from build123d import *

# Parameters (mm, degrees)
F0_W     = 14
F0_H     = 10
F0_W_2   = 6
F0_H_2   = 6
F1_DEPTH = 3
F2_DEPTH = 9


with BuildPart() as f1:
    # F0 (on Front) → F1 (new body)
    with BuildSketch(Plane.XZ):
        with Locations((-3, 0)):
            Rectangle(F0_W, F0_H)
        with Locations((-3.5, 0)):
            Rectangle(F0_W_2, F0_H_2, mode=Mode.SUBTRACT)
    extrude(amount=F1_DEPTH)

    # F0 (on Front) → F2 (join)
    with BuildSketch(Plane.XZ):
        with Locations((7, 0)):
            Rectangle(F0_W_2, F0_H)
    extrude(amount=F2_DEPTH)


solid = f1.part
Could you check a few things on this model? Use its own coordinates, in mm. A direction names the side the tool comes from. Give positions to 0.01 mm unless a question says otherwise; leave off trailing zeros. Write each loop counter-clockwise with the first axis right and the second up, starting at its lowest first coordinate (ties: lowest second). Pieces come first, ordered by that corner, then holes. Notation, with made-up numbers: (7, -18) -> (65, -18) arc R16 cw to (65, -9) -> close; hole circle Ø4 at (-36, 70). An arc over 180 degrees is marked (long way). Write each question's results on one line, items separated by ' | '. Start each with the question number.
Q1. I'm going to push flat-ended pins straight in: pin 1 Ø5 at (x, z) = (-6.5, -2.5) entering from +Y; pin 2 Ø4 at (x, y) = (-0.5, -5.5) entering from -Z; pin 3 Ø3 at (y, z) = (-7, -1.5) entering from -X. Where does each tip first touch, or does it pass through?
Q2. I need wall thicknesses on probe 1 along X at (y, z) = (-0.5, 2.75); probe 2 along X at (y, z) = (-8.5, -2.5); probe 3 along Z at (x, y) = (-4.5, -1.75). Which ranges of each line are inside material? Lowest first, please.
Q3. Suppose I cut it at D-D, the plane z = 3.5. List the corners of the cut face in (x, y) for me, and give its area (3 significant figures).
Q4. Suppose I cut it at A-A, the plane x = -3. List the corners of the cut face in (y, z) for me, and give its area (3 significant figures).
Q5. We'd pull the mould along Z, two halves only. Please class faces 4 (the face through (-6.5, -1, 0)), 5 (the face through (2, -2, 5)), 6 (the face through (-4, -1, 3)), 7 (the face through (0, 0, 0)): +Z half, -Z half, draft (parallel to the pull), parting line (faces both ways), or undercut.
Q6. Which directions (+Z, -Z, +X, -X, +Y, -Y) give clear straight access to the entire face, cutting with the end or side of a thin tool? Please do faces 1 (the face through (0, -3, 0)), 2 (the face through (-10, -1, 0)), 3 (the face through (-4, -1, -3)).
Q7. Suppose I cut it at C-C, the plane z = -2.25. List the corners of the cut face in (x, y) for me.
Q8. Suppose I cut it at B-B, the plane y = -1.5. List the corners of the cut face in (x, z) for me.
Outcome:
1) pin 1: y = 0 | pin 2: through | pin 3: x = 4
2) probe 1: -10 to -6.5, -0.5 to 10 | probe 2: 4 to 10 | probe 3: -5 to -3, 3 to 5
3) outline: (-10, -3) -> (4, -3) -> (4, -9) -> (10, -9) -> (10, 0) -> (-10, 0) -> close | area: 96.0 mm2
4) outline: (-3, -5) -> (0, -5) -> (0, -3) -> (-3, -3) -> close; (-3, 3) -> (0, 3) -> (0, 5) -> (-3, 5) -> close | area: 12.0 mm2
5) face 4: undercut | face 5: +Z half | face 6: undercut | face 7: draft
6) face 1: +Z, -Z, -X, -Y | face 2: +Z, -Z, -X, +Y, -Y | face 3: +Y, -Y
7) outline: (-10, -3) -> (-6.5, -3) -> (-6.5, 0) -> (-10, 0) -> close; (-0.5, -3) -> (4, -3) -> (4, -9) -> (10, -9) -> (10, 0) -> (-0.5, 0) -> close
8) outline: (-10, -5) -> (10, -5) -> (10, 5) -> (-10, 5) -> close; hole (-6.5, -3) -> (-0.5, -3) -> (-0.5, 3) -> (-6.5, 3) -> close
